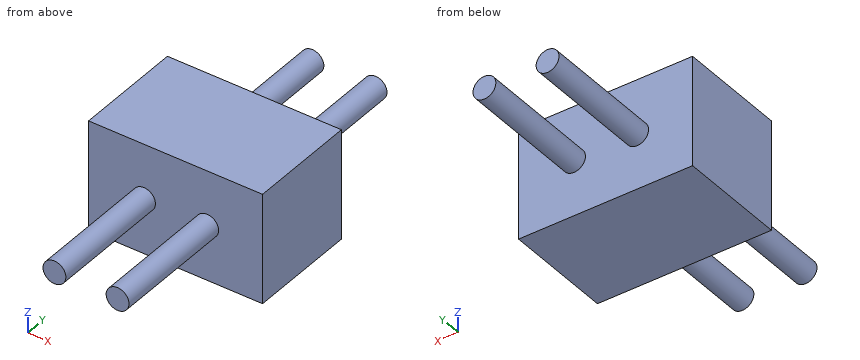
```python
from build123d import *

# Parameters (mm, degrees)
SKETCH1_W           = 3.5
SKETCH1_H           = 2.21
BOSS_EXTRUDE1_DEPTH = 2.21
SKETCH2_R           = 0.23
BOSS_EXTRUDE2_DEPTH = 2.51
BOSS_EXTRUDE3_START = 2.51
SKETCH3_R           = 0.23
BOSS_EXTRUDE3_DEPTH = 2.51


with BuildPart() as part:
    # Sketch1 → Boss-Extrude1 (new body)
    with BuildSketch(Plane(origin=(0, 0, 0), x_dir=(1, 0, 0), z_dir=(0, 1, 0))):
        with Locations((1.75, 1.105)):
            Rectangle(SKETCH1_W, SKETCH1_H)
    extrude(amount=BOSS_EXTRUDE1_DEPTH)

    # Sketch2 → Boss-Extrude2 (add)
    with BuildSketch(Plane.XZ):
        with Locations(Location((1.115, -1.105, 0), (0, 0, 270))):
            Circle(SKETCH2_R)
        with Locations(Location((2.385, -1.105, 0), (0, 0, 270))):
            Circle(SKETCH2_R)
    extrude(amount=BOSS_EXTRUDE2_DEPTH)

    # Sketch3 → Boss-Extrude3 (add)
    with BuildSketch(Plane(origin=(0, 2.21, 0), x_dir=(1, 0, 0), z_dir=(0, 1, 0)).offset(BOSS_EXTRUDE3_START)):
        with Locations(Location((2.385, 1.105, 0), (0, 0, 90))):
            Circle(SKETCH3_R)
        with Locations(Location((1.115, 1.105, 0), (0, 0, 90))):
            Circle(SKETCH3_R)
    extrude(amount=-BOSS_EXTRUDE3_DEPTH)


solid = part.part
```
Geometry check sheet. Reference: the model listing, model coordinates, mm. Round coordinates to 2 decimals unless told otherwise and drop trailing zeros. Loops run counter-clockwise (first coordinate to the right, second up) from the corner with the lowest first, then second, coordinate; pieces in that order, holes last. Notation, with made-up numbers: M -34,-26.75 L -25,-26.75 A37 cw -25,9.25 Z; hole C 60,71 d7. An arc over 180 degrees is marked long. Return JSON: item names as keys, results as strings. Group by question number.
(1) Section check C-C, the plane y = -0.75. Enter the section's corners in (x, z) (3 decimals), and give its area (3 significant figures).
(2) Section check B-B, the plane x = 0.7. Enter the section's corners in (y, z), and give its area (3 significant figures).
(3) Scan lines: line 1 along Y through (x, z) = (2.4, -1.55); line 2 along Z through (x, y) = (2.4, -1.5). Record each from-to range of solid material in increasing order. Write a range as [from, to].
(4) Section check A-A, the plane z = -0.5. Enter the section's corners in (x, y), and give its area (4 significant figures).
Data:
{
 "1": {"outline": "C 1.115,-1.105 d0.46; C 2.385,-1.105 d0.46", "area": "0.332 mm²"},
 "2": {"outline": "M 0,-2.21 L 2.21,-2.21 L 2.21,0 L 0,0 Z", "area": "4.88 mm²"},
 "3": {"line 1": "[0, 2.21]", "line 2": "[-1.33, -0.88]"},
 "4": {"outline": "M 0,0 L 3.5,0 L 3.5,2.21 L 0,2.21 Z", "area": "7.735 mm²"}
}
